Work out the finished part from the listing and answer in its coordinate system (mm). Face numbers are marked on the shaded views. A direction names the side the tool comes from. Round coordinates to 2 decimals unless told otherwise and drop trailing zeros. Order: outer loops, then holes, each group sorted by start corner. A loop starts at its lowest first (then second) coordinate and runs counter-clockwise, first axis right, second up. Notation, with made-up numbers: (39, -23.75) - (58, -23.75) arc R28 ccw to (58, 12.25) - close; hole circle Ø3 at (52, 6). An arc over 180 degrees is marked (long way). Use one line per item in the form item = value. Start each with the question number.
Q1. The part is cut by section B-B on y = -23.5. Determine the outline of the cut face in (x, z) (1 decimal).
Q2. The part is cut by section D-D on x = -1.5. Determine the outline of the cut face in (y, z), plus the area to 3 significant figures.
Q3. The part is cut by section A-A on z = 0. Determine the outline of the cut face in (x, y).
Q4. For a pull along Z with two mould halves and no side action, classify the marked faces 5, 6, 7 and 8 as +Z half, -Z half, draft (parallel to the pull), parting line (faces both ways), or undercut.
Q5. The part is cut by section C-C on z = 5. Determine the outline of the cut face in (x, y).
Q6. Which of the six approach directions +Z, -Z, +X, -X, +Y, -Y give full straight-line access (tool end or side, diameter ignored) to the marked faces 1, 2, 3 and 4?
Q7. Find the intervals of material crossed by line 1 (Z direction, x = -6.5, y = 24); line 2 (Y direction, x = -2, z = 0); line 3 (Y direction, x = -1.6, z = 0), in increasing order. Write a range as [from, to].
Q8. Given P1, Ø0.8, axis at y = -19.5, z = -9, coming from the -X side; P2, Ø6, axis at y = -23, z = 1.5, coming from the -X side; P3, Ø2.5, axis at y = 0, z = -1, coming from the +X side, each flat-ended and moving along its own axis, determine where each tip first touches the part or whether it passes through.
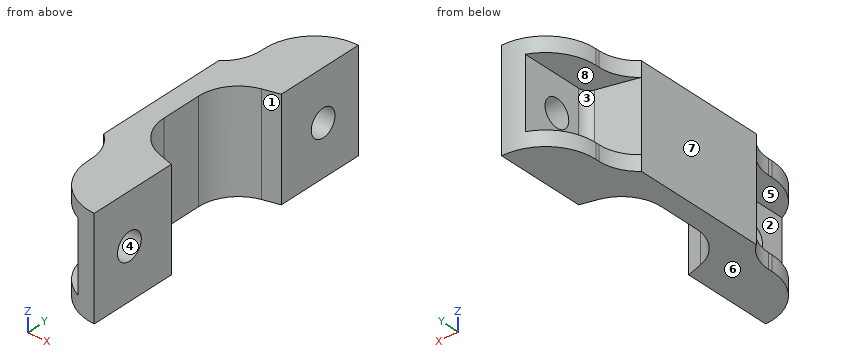
from build123d import *

# Parameters (mm, degrees)
EXTRUDE_1_DEPTH      = 10
EXTRUDE_1_DEPTH_BACK = 10
SKETCH_2_R           = 2.7
CUT_EXTRUDE_1_DEPTH  = 35.190641995
SKETCH_3_W           = 3
SKETCH_3_H           = 17.5
EXTRUDE_2_DEPTH      = 10
FILLET_1_R           = 10
FILLET_2_R           = 8
FILLET_3_R           = 8
FILLET_4_R           = 2


with BuildPart() as part:
    # 草图1 → 凸台-拉伸1 (new, two sides: drawn at the far end of the back side and taken through both)
    with BuildSketch(Plane.XY.offset(-EXTRUDE_1_DEPTH_BACK)):
        Polygon((0, 30), (0, 12.5), (-9, 10), (-9, -10), (0, -12.5), (0, -30), (-4, -30), (-4, -15.540342598), (-13, -13.040342598), (-13, 13.040342598), (-4, 15.540342598), (-4, 30), align=None)
    extrude(amount=EXTRUDE_1_DEPTH + EXTRUDE_1_DEPTH_BACK)

    # 草图2 → 切除-拉伸1 (cut, through all)
    with BuildSketch(Plane(origin=(0, 0, 0), x_dir=(0, 0, -1), z_dir=(1, 0, 0))):
        with Locations((0, 22)):
            Circle(SKETCH_2_R)
        with Locations((0, -22)):
            Circle(SKETCH_2_R)
    extrude(amount=-CUT_EXTRUDE_1_DEPTH, mode=Mode.SUBTRACT)

    # 草图3 → 凸台-拉伸2 (add)
    with BuildSketch(Plane(origin=(0, 0, 0), x_dir=(0, 0, -1), z_dir=(1, 0, 0))):
        with Locations((-8.5, 21.25)):
            Rectangle(SKETCH_3_W, SKETCH_3_H)
        with Locations((8.5, 21.25)):
            Rectangle(SKETCH_3_W, SKETCH_3_H)
        with Locations((-8.5, -21.25)):
            Rectangle(SKETCH_3_W, SKETCH_3_H)
        with Locations((8.5, -21.25)):
            Rectangle(SKETCH_3_W, SKETCH_3_H)
    extrude(amount=-EXTRUDE_2_DEPTH)

    # 圆角1
    # the kernel refuses this fillet: 10 mm, written as the material it takes off along each edge
    with BuildSketch(Plane(origin=(-10, -30, -35), x_dir=(1, 0, 0), z_dir=(0, 0, 1)), Plane(origin=(-10, 30, -35), x_dir=(0, -1, 0), z_dir=(0, 0, 1))) as fillet_1_piece_1:
        with BuildLine():
            CenterArc((FILLET_1_R, FILLET_1_R), FILLET_1_R, 180, 90)
            Line((0, FILLET_1_R), (0, 0))
            Line((0, 0), (FILLET_1_R, 0))
        make_face()
    extrude(amount=53, mode=Mode.SUBTRACT)

    # 圆角2
    # the kernel refuses this fillet: 8 mm, written as the material it adds along each edge
    with BuildSketch(Plane(origin=(-10, 13.873675932, 7), x_dir=(0, 1, 0), z_dir=(0, 0, 1))) as fillet_2_piece_1:
        with BuildLine():
            CenterArc((5.411664665, 8), FILLET_2_R, 218.682187453, 51.317812547)
            Line((-0.833333333, 3), (-0.958233293, 2.9))
            ThreePointArc((-0.958233293, 2.9), (-0.570829532, 1.457176982), (-0.154162866, -0.042823018))
            Line((-0.154162866, -0.042823018), (0, -0.16))
            Line((0, -0.16), (5.411664665, -0.16))
            Line((5.411664665, -0.16), (5.411664665, 0))
        make_face()
    extrude(amount=3)
    with BuildSketch(Plane(origin=(-10, 13.873675932, -7), x_dir=(-0.963517909629979, -0.26764386378595645, 0), z_dir=(0, 0, -1)), Plane(origin=(-10, -13.873675932, 7), x_dir=(-0.963517909629979, 0.26764386378595645, 0), z_dir=(0, 0, 1))) as fillet_2_piece_2:
        with BuildLine():
            CenterArc((6.259744437, 7.355386736), FILLET_2_R, 195.524110997, 51.317812547)
            Line((-1.44839884, 5.214235826), (-1.602561706, 5.171412807))
            Line((-1.602561706, 5.171412807), (-0.154162866, -0.042823018))
            Line((-0.154162866, -0.042823018), (0, -0.16))
            ThreePointArc((0, -0.16), (1.556795141, -0.16), (3.050667199, -0.147107735))
            Line((3.050667199, -0.147107735), (3.113590282, 0))
        make_face()
    extrude(amount=3)
    with BuildSketch(Plane(origin=(-10, -13.873675932, -7), x_dir=(-0.963517909629979, 0.26764386378595645, 0), z_dir=(0, 0, -1))) as fillet_2_piece_3:
        with BuildLine():
            CenterArc((6.259744437, -7.355386736), FILLET_2_R, 113.158076457, 51.317812547)
            Line((-1.44839884, -5.214235826), (-1.602561706, -5.171412807))
            Line((-1.602561706, -5.171412807), (-0.154162866, 0.042823018))
            Line((-0.154162866, 0.042823018), (0, 0.16))
            ThreePointArc((0, 0.16), (1.556795141, 0.16), (3.050667199, 0.147107735))
            Line((3.050667199, 0.147107735), (3.113590282, 0))
        make_face()
    extrude(amount=3)

    # 圆角3
    fillet_3_edges = [part.edges().sort_by_distance(p)[0] for p in [
        (-9, 10, 0),
        (-9, -10, 0),
    ]]
    fillet(fillet_3_edges, radius=FILLET_3_R)

    # 圆角4
    fillet_4_edges = [part.edges().sort_by_distance(p)[0] for p in [
        (-4, 15.540342598, 0),
        (-4, -15.540342598, 0),
    ]]
    fillet(fillet_4_edges, radius=FILLET_4_R)


solid = part.part
Found:
q1.outline = (-9.4, -10) - (0, -10) - (0, -2.2) - (-4, -2.2) - (-4, -7) - (-9.4, -7) - close; (-9.4, 7) - (-4, 7) - (-4, 2.2) - (0, 2.2) - (0, 10) - (-9.4, 10) - close
q2.outline = (-29.89, -10) - (-12.08, -10) - (-12.08, 10) - (-29.89, 10) - close; (12.08, -10) - (29.89, -10) - (29.89, 10) - (12.08, 10) - close; hole circle Ø5.4 at (-22, 0); hole circle Ø5.4 at (22, 0)
q2.area = 666 mm²
q3.outline = (-13, -13.04) - (-5.46, -15.13) arc R2 cw to (-4, -17.06) - (-4, -19.3) - (0, -19.3) - (0, -12.5) - (-3.14, -11.63) arc R8 cw to (-9, -3.92) - (-9, 3.92) arc R8 cw to (-3.14, 11.63) - (0, 12.5) - (0, 19.3) - (-4, 19.3) - (-4, 17.06) arc R2 cw to (-5.46, 15.13) - (-13, 13.04) - close; (-4, -29.17) arc R10 ccw to (0, -30) - (0, -24.7) - (-4, -24.7) - close; (-4, 24.7) - (0, 24.7) - (0, 30) arc R10 ccw to (-4, 29.17) - close
q4.face_5 = undercut
q4.face_6 = -Z half
q4.face_7 = draft
q4.face_8 = undercut
q5.outline = (-13, -13.04) - (-5.46, -15.13) arc R2 cw to (-4, -17.06) - (-4, -29.17) arc R10 ccw to (0, -30) - (0, -12.5) - (-3.14, -11.63) arc R8 cw to (-9, -3.92) - (-9, 3.92) arc R8 cw to (-3.14, 11.63) - (0, 12.5) - (0, 30) arc R10 ccw to (-4, 29.17) - (-4, 17.06) arc R2 cw to (-5.46, 15.13) - (-13, 13.04) - close
q6.face_1 = +Z, -Z, +X
q6.face_2 = -X, -Y
q6.face_3 = -X, +Y
q6.face_4 = +X, -X
q7.line_1 = [-10, -7], [7, 10]
q7.line_2 = [-29.8, -24.7], [-19.3, -11.94], [11.94, 19.3], [24.7, 29.8]
q7.line_3 = [-29.87, -24.7], [-19.3, -12.06], [12.06, 19.3], [24.7, 29.87]
q8.P1 = -10
q8.P2 = -4
q8.P3 = -9
